Verification items for this drawing (mm, ordinates from the low corner). Coordinates: 2 decimals unless noted, no trailing zeros. Loops run counter-clockwise (first coordinate to the right, second up) from the corner with the lowest first, then second, coordinate; pieces in that order, holes last. Notation, with made-up numbers: (58.25, -10.5) - (71.25, -10.5) arc R16 ccw to (71.25, -0.5) - close; hole circle Ø4 at (-29.5, 10). An arc over 180 degrees is marked (long way). One line per item, written item: value. Start each with the question number.
(1) Section check A-A (x = 105.1). Record the boundary of the cut face in (y, z), plus the area to 3 significant figures.
(2) Thickness scan on probe 1 along X at (y, z) = (2.9, 56.5); probe 2 along X at (y, z) = (4.05, 143); probe 3 along Z at (x, y) = (107, 2.95) (1 decimal). Record the ranges inside material, lowest first. Write a range as [from, to].
(3) Section check B-B (z = 53.5). Record the boundary of the cut face in (x, y).
(4) Section check C-C (y = 1.8). Record the boundary of the cut face in (x, z), plus the area to 3 significant figures.
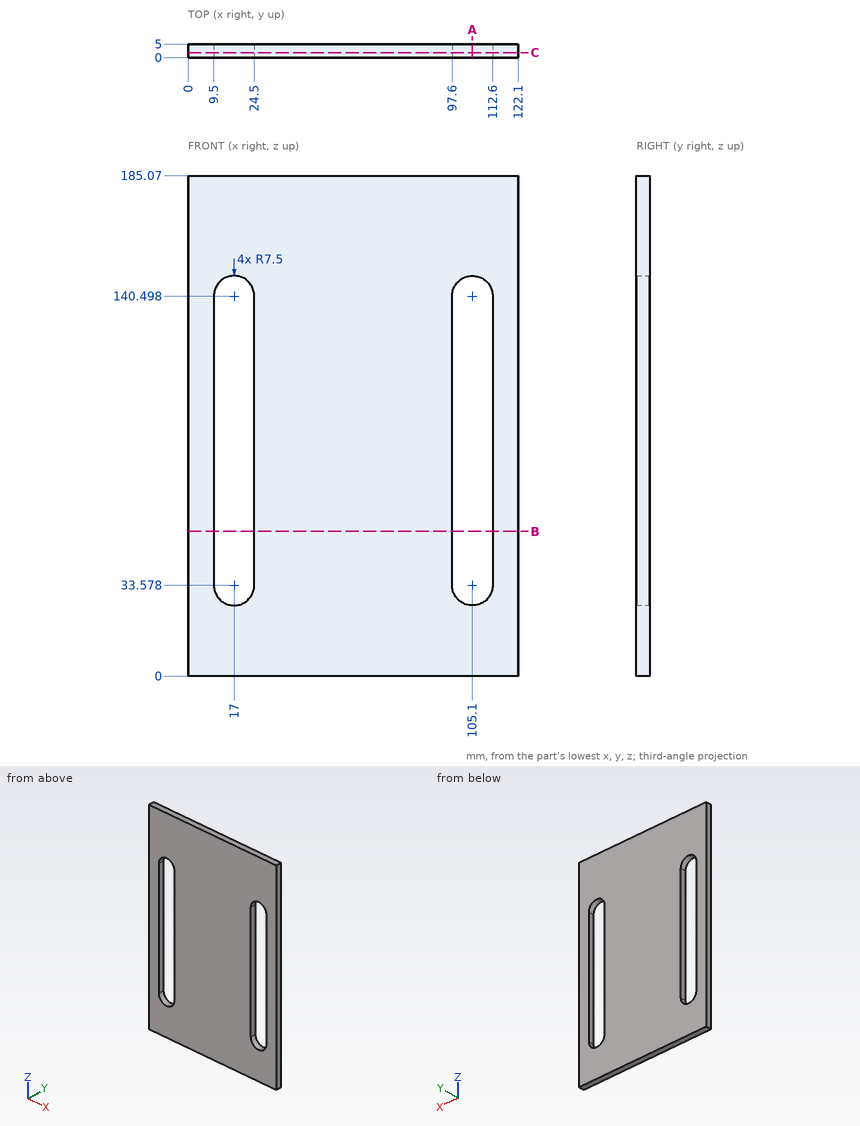
Responses:
1. outline: (0, 0) - (5, 0) - (5, 26.08) - (0, 26.08) - close; (0, 148) - (5, 148) - (5, 185.07) - (0, 185.07) - close
1. area: 316 mm²
2. probe 1: x = [0, 9.5], [24.5, 97.6], [112.6, 122.1]
2. probe 2: x = [0, 9.93], [24.07, 98.03], [112.17, 122.1]
2. probe 3: z = [0, 26.3], [147.8, 185.1]
3. outline: (0, 0) - (9.5, 0) - (9.5, 5) - (0, 5) - close; (24.5, 0) - (97.6, 0) - (97.6, 5) - (24.5, 5) - close; (112.6, 0) - (122.1, 0) - (122.1, 5) - (112.6, 5) - close
4. outline: (0, 0) - (122.1, 0) - (122.1, 185.07) - (0, 185.07) - close; hole (9.5, 33.58) arc R7.5 ccw to (24.5, 33.58) - (24.5, 140.5) arc R7.5 ccw to (9.5, 140.5) - close; hole (97.6, 33.58) arc R7.5 ccw to (112.6, 33.58) - (112.6, 140.5) arc R7.5 ccw to (97.6, 140.5) - close
4. area: 19,000 mm²
